```python
from build123d import *

# Parameters (mm, degrees)
SKETCH1_W           = 393.4
SKETCH1_H           = 185.491905347
BOSS_EXTRUDE1_DEPTH = 3.3
SKETCH2_R           = 2.00000001
SKETCH2_R_2         = 2
CUT_EXTRUDE1_DEPTH  = 4
SKETCH3_W           = 169.7
SKETCH3_H           = 21.4
CUT_EXTRUDE2_DEPTH  = 6
SKETCH4_R           = 2
CUT_EXTRUDE3_DEPTH  = 276.628325081


with BuildPart() as part:
    # Sketch1 → Boss-Extrude1 (new body)
    with BuildSketch(Plane.XY):
        with Locations((27, 68.245952673)):
            Rectangle(SKETCH1_W, SKETCH1_H)
    extrude(amount=BOSS_EXTRUDE1_DEPTH)

    # Sketch2 → Cut-Extrude1 (cut)
    with BuildSketch(Plane(origin=(0, 0, 0), x_dir=(-1, 0, 0), z_dir=(0, 0, -1))):
        with Locations((-27, 40.495952673)):
            Circle(SKETCH2_R)
        with Locations((-27, 120.495952673)):
            Circle(SKETCH2_R)
        with Locations((-188.85, 2.5)):
            Circle(SKETCH2_R_2)
        with Locations((-88.85, 2.5)):
            Circle(SKETCH2_R_2)
        with Locations((34.85, 2.5)):
            Circle(SKETCH2_R_2)
        with Locations((134.85, 2.5)):
            Circle(SKETCH2_R_2)
    extrude(amount=-CUT_EXTRUDE1_DEPTH, mode=Mode.SUBTRACT)

    # Sketch3 → Cut-Extrude2 (cut)
    with BuildSketch(Plane(origin=(0, 0, 0), x_dir=(-1, 0, 0), z_dir=(0, 0, -1))):
        with Locations((84.85, 75.5)):
            Rectangle(SKETCH3_W, SKETCH3_H)
        with Locations((-138.85, 75.5)):
            Rectangle(SKETCH3_W, SKETCH3_H)
    extrude(amount=-CUT_EXTRUDE2_DEPTH, mode=Mode.SUBTRACT)

    # Sketch4 → Cut-Extrude3 (cut, through all)
    with BuildSketch(Plane.XY.offset(3.3)):
        with Locations((93.303368669, 91.2)):
            Circle(SKETCH4_R)
        with Locations((73.303368669, 91.2)):
            Circle(SKETCH4_R)
        with Locations((181.525840122, 59.8)):
            Circle(SKETCH4_R)
        with Locations((201.525840122, 59.8)):
            Circle(SKETCH4_R)
        with Locations((-127.525840122, 93.7)):
            Circle(SKETCH4_R)
        with Locations((-147.525840122, 93.7)):
            Circle(SKETCH4_R)
        with Locations((-19.303368669, 57.3)):
            Circle(SKETCH4_R)
        with Locations((-39.303368669, 57.3)):
            Circle(SKETCH4_R)
    extrude(amount=-CUT_EXTRUDE3_DEPTH, mode=Mode.SUBTRACT)


solid = part.part
```
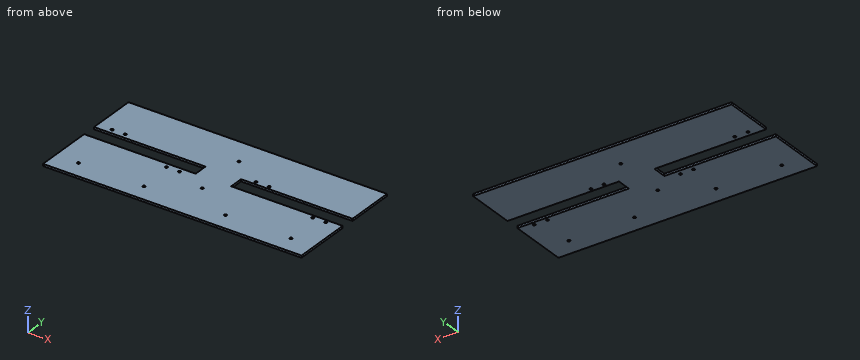
CAD build for the part. Positions are in the model's coordinates, mm. Round coordinates to 2 decimals unless told otherwise and drop trailing zeros. Write each loop counter-clockwise with the first axis right and the second up, starting at its lowest first coordinate (ties: lowest second). Pieces come first, ordered by that corner, then holes.
Item 1: Band-saw the part on A-A on x = 125. Write the cut outline in (y, z), then the cut area to 3 significant figures.
Filled in:
outline: (-24.5, 0) - (64.8, 0) - (64.8, 3.3) - (-24.5, 3.3) - close; (86.2, 0) - (160.99, 0) - (160.99, 3.3) - (86.2, 3.3) - close
area: 542 mm2
Item 2: Drill centre lines: L1, parallel to Y at x = 188.85, z = 1.45; L2, parallel to Y at x = 182.5, z = 0.6; L3, parallel to Y at x = -102, z = 2.5. Where is each one in solid material? Low to high.
Filled in:
L1: y = -24.5 to 0.5, 4.5 to 64.8, 86.2 to 160.99
L2: y = -24.5 to 58.05, 61.55 to 64.8, 86.2 to 160.99
L3: y = -24.5 to 64.8, 86.2 to 160.99
Item 3: Band-saw the part on B-B on z = 1.3. Give the number of separate pieces and of enclosed holes in the cut face, then the cut area to 3 significant figures.
Filled in:
separate pieces: 1
enclosed holes: 14
area: 65,500 mm2
Item 4: Drop a flat-ended pin along its axis: pin 1 Ø3.5 at (x, y) = (188.85, 2.5) entering from +Z. Give the stop position or say it passes through.
Filled in:
pin 1: passes through
